```python
from build123d import *

# Parameters (mm, degrees)
F1_DEPTH = 9.525
F2_R     = 4.76249


# Not quite as in the source:
# - a fillet or chamfer is up to 0.001 mm smaller than in the source, because OpenCascade refuses the exact size


with BuildPart() as f1:
    # F0 (on Front) → F1 (new body)
    with BuildSketch(Plane.XZ):
        Polygon((-9.3524411189, 93.575365177), (-9.3524411189, -58.8385015355), (-4.5891202249, -58.8385015355), (0.174200669, -58.8385015355), (0.174200669, 93.575365177), (170.0456099196, 93.575365177), (170.0456099196, 404.7306356684), (160.5287608864, 404.7306356684), (160.5287608864, 103.1056356684), (-4.5891202249, 103.1056356684), (-169.7070013363, 103.1056356684), (-169.7070013363, 404.7306356684), (-179.2238503695, 404.7306356684), (-179.2238503695, 93.575365177), align=None)
    extrude(amount=F1_DEPTH)

    # F2 (radius 4.7625 in the source; OpenCascade refuses exactly that, so slightly less here)
    f2_edges = [f1.edges().sort_by_distance(p)[0] for p in [
        (170.04561, -9.525, 249.153),
        (170.04561, 0, 249.153),
        (-4.58912, 0, 103.105636),
        (-4.58912, -9.525, 103.105636),
        (-94.288146, -9.525, 93.575365),
        (-94.288146, 0, 93.575365),
        (85.109905, -9.525, 93.575365),
        (85.109905, 0, 93.575365),
        (0.174201, -9.525, 17.368432),
        (-9.352441, -9.525, 17.368432),
        (-9.352441, 0, 17.368432),
        (0.174201, 0, 17.368432),
        (-179.22385, 0, 249.153),
        (-179.22385, -9.525, 249.153),
    ]]
    fillet(f2_edges, radius=F2_R)


solid = f1.part
```
Check sheet for the modelled part. Datum: model origin and axes. Units: mm. Give positions to 0.01 mm unless a question says otherwise; leave off trailing zeros. Order: outer loops, then holes, each group sorted by start corner. A loop starts at its lowest first (then second) coordinate and runs counter-clockwise, first axis right, second up. Notation, with made-up numbers: M 82,53.25 L 108,53.25 A18 cw 108,60.25 Z; hole C -26.5,67 d2. An arc over 180 degrees is marked long. Answer in a Markdown table with one row per item.
1) Gauge pin test, flat ends, axial feed: P1, Ø4, axis at y = -4.5, z = 14.5, coming from the +X side; P2, Ø2, axis at y = -1, z = 314, coming from the +X side; P3, Ø5, axis at x = -139, y = -8.5, coming from the +Z side. Record the tip position at first contact, or that the pin passes through.
Filled sheet:
| item | result |
|---|---|
| P1 | stops at x = 0.17 |
| P2 | stops at x = 169.16 |
| P3 | stops at z = 102.94 |
2) Thickness scan on L1, parallel to X at y = -5, z = 168.5; L2, parallel to X at y = -5.25, z = 7; L3, parallel to Z at x = 96, y = -4.75. Record the ranges inside material, lowest first. Write a range as [from, to].
Filled sheet:
| item | result |
|---|---|
| L1 | x = [-179.22, -169.71], [160.53, 170.04] |
| L2 | x = [-9.33, 0.15] |
| L3 | z = [93.58, 103.11] |
3) Release check for a two-part mould opening along X. For faces 1 (the flat face through (-169.707, -5, 249)), 2 (the flat face through (165, -5, 404.731)) record: +X half, -X half, draft (parallel to the pull), parting line (faces both ways), or undercut.
Filled sheet:
| item | result |
|---|---|
| face 1 | undercut |
| face 2 | draft |
4) Cross-section at D-D, the plane y = -8. Enter the section's corners in (x, z) (1 decimal).
Filled sheet:
| item | result |
|---|---|
| outline | M -178,94.8 L -8.1,94.8 L -8.1,-58.8 L -1.1,-58.8 L -1.1,94.8 L 168.8,94.8 L 168.8,404.7 L 160.5,404.7 L 160.5,101.8 L -169.7,101.8 L -169.7,404.7 L -178,404.7 Z |
